For this review, take the finished solid that the model builds, in its own axes (mm). A direction names the side the tool comes from. Coordinates: 2 decimals unless noted, no trailing zeros. Order: outer loops, then holes, each group sorted by start corner. A loop starts at its lowest first (then second) coordinate and runs counter-clockwise, first axis right, second up. Notation, with made-up numbers: (52, 53.5) -> (82, 53.5) arc R30 cw to (82, 86.5) -> close; hole circle Ø1 at (-35, 61.25). An arc over 180 degrees is marked (long way). Return JSON: item names as keys, results as strings. Group by question number.
Item 1: For line 1 along Z through (x, y) = (21, 1.8); line 2 along X through (y, z) = (2.8, -31), list the stretches that pass through material, from the lowest coordinate up.
Item 2: Machinability: for faces 1 (the flat face through (-50.378, 2, 17)), 2 (the flat face through (17.872, 2, -31)), 3 (the flat face through (-35, 2, -14.769)), which of the approach directions +Z, -Z, +X, -X, +Y, -Y give a long, thin tool a straight path to every point of the face, cutting with its end or side? Answer none if there is none.
Item 3: Take a section at C-C (z = -28). Write out the cut boundary in (x, y), then the cut area to 3 significant figures.
Item 4: Insertion check: pin 1 (1.2 mm diameter, centred on y = 2.5, z = -30, fed in from +X). The pin has a flat end and moves straight along its axis. Give the tip position at first contact, or say it passes through.
Item 5: Take a section at B-B (x = 20). Write out the cut boundary in (y, z).
Item 6: Take a section at A-A (y = 1.1). Write out the cut boundary in (x, z).
Autodesk Inventor part; units mm, degrees
ref_plane "YZ Plane" through (0, 0, 0) normal (1, 0, 0) x (0, 1, 0)
ref_plane "XZ Plane" through (0, 0, 0) normal (0, 1, 0) x (-1, 0, 0)
ref_plane "XY Plane" through (0, 0, 0) normal (0, 0, 1) x (1, 0, 0)
sketch "Sketch1" plane through (0, 0, 0) normal (0, 1, 0) x (-1, 0, 0)
  line L0 (-49.6221, -50.9693) -> (50.3779, -50.9693)
  line L1 (50.3779, -50.9693) -> (50.3779, 49.0307)
  line L2 (50.3779, 49.0307) -> (-49.6221, 49.0307)
  line L3 (-49.6221, 49.0307) -> (-49.6221, -50.9693)
  line L4 (-17.8721, -0.5117) -> (18.6279, -0.5117)
  line L5 (18.6279, -0.5117) -> (18.6279, -50.9693)
  line L6 (18.6279, -50.9693) -> (-17.8721, -50.9693)
  line L7 (-17.8721, -50.9693) -> (-17.8721, -0.5117)
  line L8 (-49.6221, -18.7693) -> (50.3779, -18.7693)
  line L9 (50.3779, -18.7693) -> (50.3779, -50.9693)
  line L10 (50.3779, -50.9693) -> (-49.6221, -50.9693)
  line L11 (-49.6221, -50.9693) -> (-49.6221, -18.7693)
  line L12 (-49.6221, -18.7693) -> (50.3779, -18.7693)
  line L13 (50.3779, -18.7693) -> (50.3779, -14.7693)
  line L14 (50.3779, -14.7693) -> (-49.6221, -14.7693)
  line L15 (-49.6221, -14.7693) -> (-49.6221, -18.7693)
  line L16 (-49.6221, -34.8693) -> (50.3779, -34.8693)
  line L17 (-49.6221, -50.9693) -> (50.3779, -50.9693)
  line L18 (50.3779, -50.9693) -> (50.3779, -46.9693)
  line L19 (50.3779, -46.9693) -> (-49.6221, -46.9693)
  line L20 (-49.6221, -46.9693) -> (-49.6221, -50.9693)
  point P0 (0, 0)
  point P1 (0.3779, -50.9693)
  point P2 (0.3779, -50.9693)
  point P3 (0.3779, -50.9693)
  point P4 (-49.6221, -14.7693)
  point P5 (-17.8721, -14.7693)
  point P6 (-17.8721, -46.9693)
  point P7 (18.6279, -46.9693)
  point P8 (18.6279, -14.7693)
  dimension "d0" = 100
  dimension "d1" = 100
  dimension "d2" = 36.5
  dimension "d3" = 100
  dimension "d4" = 32.2
  dimension "d5" = 4
  dimension "d6" = 4
extrude "Extrusion1" add sketch "Sketch1" along normal blind 4 contours L7 L16 L5 L19 | L7 L8 L5 L16 | L7 L14 L5 L8 | L3 L2 L1 L14 L5 L4 L7 | L7 L4 L5 L14
properties part number "podstawa"
Findings below:
{
 "1": {"line 1": "z = -14.77 to 49.03", "line 2": "x = -18.63 to 17.87"},
 "2": {"face 1": "+Z, -Z, -X, +Y, -Y", "face 2": "-Z, +X, +Y, -Y", "face 3": "-Z, -X, +Y, -Y"},
 "3": {"outline": "(-18.63, 0) -> (17.87, 0) -> (17.87, 4) -> (-18.63, 4) -> close", "area": "146 mm2"},
 "4": {"pin 1": "stops at x = 17.87"},
 "5": {"outline": "(0, -14.77) -> (4, -14.77) -> (4, 49.03) -> (0, 49.03) -> close"},
 "6": {"outline": "(-50.38, -14.77) -> (-18.63, -14.77) -> (-18.63, -46.97) -> (17.87, -46.97) -> (17.87, -14.77) -> (49.62, -14.77) -> (49.62, 49.03) -> (-50.38, 49.03) -> close"}
}
